Check sheet for the modelled part. Datum: model origin and axes. Units: mm. A direction names the side the tool comes from. Coordinates: 2 decimals unless noted, no trailing zeros. Write each loop counter-clockwise with the first axis right and the second up, starting at its lowest first coordinate (ties: lowest second). Pieces come first, ordered by that corner, then holes. Notation, with made-up numbers: (15, 9) -> (23, 9) arc R20 ccw to (23, 29) -> close; hole circle Ø5 at (74, 77.5). An arc over 180 degrees is marked (long way). Put each result on its own line as item: value.
```python
from build123d import *
from build123d.topology import SkipClean

# Parameters (mm, degrees)
SKETCH2_W           = 50.8
SKETCH2_H           = 50.8
SKETCH2_R           = 7.62
SKETCH2_R_2         = 2.4765
BOSS_EXTRUDE1_DEPTH = 6.35
SKETCH3_W           = 44.45
SKETCH3_H           = 50.8
SKETCH3_R           = 6.35
BOSS_EXTRUDE2_DEPTH = 12.7
SKETCH9_R           = 12.7
CUT_EXTRUDE2_DEPTH  = 10.16
RIB8_REACH          = 86.481
SKETCH13_WALL_W     = 234.462510634
SKETCH13_WALL_H     = 3.175
RIB9_START          = -3.175
RIB9_DEPTH          = 3.175
BOSS_EXTRUDE5_REACH = 73.113
FILLET2_R           = 4.7625
SKETCH22_W          = 44.45
SKETCH22_H          = 50.8
BOSS_EXTRUDE6_DEPTH = 25.4
SKETCH20_R          = 6.477
CUT_EXTRUDE3_DEPTH  = 50.8
SKETCH23_R          = 19.177
CUT_EXTRUDE4_DEPTH  = 15.494
BOSS_EXTRUDE7_START = 6.35
SKETCH25_W          = 88.9
SKETCH25_H          = 50.8
SKETCH25_R          = 2.4765
SKETCH25_R_2        = 7.62
BOSS_EXTRUDE7_DEPTH = 6.35


# Read off the part's stored shape, not the designer's step: Rib9
with BuildPart() as part:
    # Sketch2 → Boss-Extrude1 (new body)
    with BuildSketch(Plane(origin=(0, 0, 0), x_dir=(0, 0, -1), z_dir=(1, 0, 0))):
        with Locations((25.4, 0)):
            Rectangle(SKETCH2_W, SKETCH2_H)
        with Locations((25.4, 0)):
            Circle(SKETCH2_R, mode=Mode.SUBTRACT)
        with Locations((32.732348419, 12.7)):
            Circle(SKETCH2_R_2, mode=Mode.SUBTRACT)
        with Locations((32.732348419, -12.7)):
            Circle(SKETCH2_R_2, mode=Mode.SUBTRACT)
        with Locations((10.735303163, 0)):
            Circle(SKETCH2_R_2, mode=Mode.SUBTRACT)
    extrude(amount=BOSS_EXTRUDE1_DEPTH)

    # Sketch3 → Boss-Extrude2 (add)
    with BuildSketch(Plane.XY):
        with Locations((22.225, 0)):
            Rectangle(SKETCH3_W, SKETCH3_H)
        with Locations((25.4, 0)):
            Circle(SKETCH3_R, mode=Mode.SUBTRACT)
    extrude(amount=BOSS_EXTRUDE2_DEPTH)

    # Sketch9 → Cut-Extrude2 (cut)
    with BuildSketch(Plane(origin=(0, 0, 0), x_dir=(-1, 0, 0), z_dir=(0, 0, -1))):
        with Locations((-25.4, 0)):
            Circle(SKETCH9_R)
    extrude(amount=-CUT_EXTRUDE2_DEPTH, mode=Mode.SUBTRACT)

    # Sketch13 wall → Rib8 (add, up to next)
    with BuildSketch(Plane(origin=(25.4, 25.4, -25.4), x_dir=(-0.6, 0, -0.8), z_dir=(-0.8, 0, 0.6)), mode=Mode.PRIVATE) as rib8_sk1:
        with Locations((0, 1.5875)):
            Rectangle(SKETCH13_WALL_W, SKETCH13_WALL_H)
    rib8_tool1 = extrude(rib8_sk1.sketch, amount=RIB8_REACH, mode=Mode.PRIVATE) - part.part
    add(rib8_tool1.solids().sort_by_distance((25.4, 25.4, -25.4))[0])

    # Rib9 outline → Rib9 (add)
    with BuildSketch(Plane(origin=(0, -25.4, 0), x_dir=(-1, 0, 0), z_dir=(0, -1, 0)).offset(RIB9_START)):
        Polygon((-6.35, 50.8), (-44.45, 0), (-6.35, 0), align=None)
    extrude(amount=RIB9_DEPTH)

    # Sketch17 → Boss-Extrude5 (add, up to next)
    with BuildSketch(Plane(origin=(1.058333333, 1.058333333, -1.058333333), x_dir=(0.8164965809277261, -0.408248290463863, 0.408248290463863), z_dir=(-0.5773502691896257, -0.5773502691896258, 0.5773502691896258)), mode=Mode.PRIVATE) as boss_extrude5_sk1:
        Polygon((6.480941611, -29.185832393), (6.480941611, -2.24506403), (29.812331411, -15.715448212), align=None)
    boss_extrude5_tool1 = extrude(boss_extrude5_sk1.sketch, amount=BOSS_EXTRUDE5_REACH, mode=Mode.PRIVATE) - part.part
    boss_extrude5 = boss_extrude5_tool1.solids().sort_by_distance((12.7, -15.875, -6.35))[0]
    add(boss_extrude5)

    # Mirror1: Boss-Extrude5 across plane
    add(boss_extrude5.mirror(Plane.ZX))

    # Fillet2
    fillet2_edges = [part.edges().sort_by_distance(p)[0] for p in [
        (6.35, 0, 0),
        (15.875, 22.225, -9.525),
        (15.875, 12.7, 0),
        (6.35, 12.7, -9.525),
        (6.35, 22.225, -34.925),
        (34.925, 22.225, 0),
        (6.35, -22.225, -34.925),
        (34.925, -22.225, 0),
        (6.35, -12.7, -9.525),
        (15.875, -12.7, 0),
        (15.875, -22.225, -9.525),
    ]]
    fillet(fillet2_edges, radius=FILLET2_R)

    # Sketch22 → Boss-Extrude6 (add)
    with BuildSketch(Plane.XY.offset(12.7)):
        with Locations((22.225, 0)):
            Rectangle(SKETCH22_W, SKETCH22_H)
    extrude(amount=BOSS_EXTRUDE6_DEPTH)

    # Sketch20 → Cut-Extrude3 (cut)
    with BuildSketch(Plane.XY.offset(12.7)):
        with Locations(Location((25.4, 0, 0), (0, 0, 180))):
            Circle(SKETCH20_R)
    extrude(amount=CUT_EXTRUDE3_DEPTH, mode=Mode.SUBTRACT)

    # Sketch23 → Cut-Extrude4 (cut)
    with BuildSketch(Plane(origin=(6.35, 0, 0), x_dir=(0, 0, -1), z_dir=(1, 0, 0))):
        with Locations((25.4, 0)):
            Circle(SKETCH23_R)
    extrude(amount=CUT_EXTRUDE4_DEPTH, mode=Mode.SUBTRACT)

    # Sketch25 → Boss-Extrude7 (add)
    with SkipClean():  # the faces are left unmerged after this step: merging them gives an invalid solid
        with BuildSketch(Plane.ZY.offset(BOSS_EXTRUDE7_START)):
            with Locations((-6.35, 0)):
                Rectangle(SKETCH25_W, SKETCH25_H)
            with Locations((-32.732348419, -12.7)):
                Circle(SKETCH25_R, mode=Mode.SUBTRACT)
            with Locations((-10.735303163, 0)):
                Circle(SKETCH25_R, mode=Mode.SUBTRACT)
            with Locations((-32.732348419, 12.7)):
                Circle(SKETCH25_R, mode=Mode.SUBTRACT)
            with Locations((-25.4, 0)):
                Circle(SKETCH25_R_2, mode=Mode.SUBTRACT)
        extrude(amount=-BOSS_EXTRUDE7_DEPTH)


solid = part.part
```
Q1. Tool access check on faces 5 (the flat face through (13.514, 16.191, -5.852)), 6 (the cylindrical face through (31.87, -0.28, 25.22)), 7 (the flat face through (-6.35, 0, -7)), 8 (the cylindrical face through (13.286, 3.815, 5.009)), 9 (the flat face through (44.45, 0, 19)). Record the directions out of +Z, -Z, +X, -X, +Y, -Y that give a thin tool (end or side, any length) a straight path to the whole face; none if there is none.
Recorded:
face 5: -Z, +X
face 6: +Z
face 7: +Z, -Z, -X, +Y, -Y
face 8: -Z
face 9: +Z, -Z, +X, +Y, -Y
Q2. Cross-section at C-C (y = -3.5). State how many separate pieces and enclosed holes the cut face has, plus the area to 3 significant figures.
Recorded:
separate pieces: 3
enclosed holes: 0
area: 1,860 mm2
Q3. Cross-section at D-D (x = 1). Record the cut outline in (y, z).
Recorded:
outline: (-25.4, -50.8) -> (25.4, -50.8) -> (25.4, 38.1) -> (-25.4, 38.1) -> close; hole circle Ø4.95 at (-12.7, -32.73); hole circle Ø15.24 at (0, -25.4); hole circle Ø4.95 at (0, -10.74); hole circle Ø4.95 at (12.7, -32.73)
Q4. Material ranges on line 1 along Z through (x, y) = (-2, 0); line 2 along Y through (x, z) = (37, -8) (3 decimals); line 3 along Z through (x, y) = (2.5, 12.7), recorded low to high.
Recorded:
line 1: z = -50.8 to -33.02, -17.78 to -13.21, -8.26 to 38.1
line 2: y = -25.4 to -22.225, 22.225 to 25.4
line 3: z = -50.8 to -35.21, -30.26 to 38.1
Q5. Depth check by flat-ended pin: P1, Ø6.5, axis at y = 0, z = -10.74, coming from the +X side; P2, Ø12.5, axis at x = 24.5, y = 0, coming from the -Z side. Enter the tip coordinate at first touch or a pass-through.
Recorded:
P1: stops at x = 6.35
P2: stops at z = 10.16
Q6. Mould release check, pull along Y, two halves, no side actions. Record for faces 1 (the flat face through (25.7, 24, -25)), 2 (the flat face through (13, -25.4, 3)), 3 (the cylindrical face through (7.71, 0.06, -1.43)), 4 (the cylindrical face through (7.156, 12.741, -9.302)): released by +Y, released by -Y, zero draft, split by the parting line, or undercut.
Recorded:
face 1: zero draft
face 2: released by -Y
face 3: undercut
face 4: undercut
